CAD build for the part. Positions are in the model's coordinates, mm. Face numbers are marked on the shaded views. A direction names the side the tool comes from. Give positions to 0.01 mm unless a question says otherwise; leave off trailing zeros. Loops run counter-clockwise (first coordinate to the right, second up) from the corner with the lowest first, then second, coordinate; pieces in that order, holes last. Notation, with made-up numbers: M -21,63 L -17,63 A24 ccw -17,96 Z; hole C 70.25,-22 d3. An arc over 180 degrees is marked long. Answer as CSV lines item,"result".
from build123d import *

# Parameters (mm, degrees)
F1_DEPTH = 63.5
F2_DEPTH = 25.4
F3_DEPTH = 7.9375
F5_R     = 6.35


with BuildPart() as f1:
    # F0 (on Front) → F1 (new body, symmetric)
    with BuildSketch(Plane.XZ):
        Polygon((-46.0913150109, 34.0935156439), (-46.0913150109, 15.0435156439), (36.4586849891, 15.0435156439), (36.4586849891, 34.0935156439), (17.4086849891, 34.0935156439), align=None)
    extrude(amount=F1_DEPTH, both=True)

    # F0 (on Front) → F2 (join, symmetric)
    with BuildSketch(Plane.XZ):
        with BuildLine():
            Line((17.4086849891, 34.0935156439), (36.4586849891, 34.0935156439))
            Line((36.4586849891, 34.0935156439), (36.4586849891, 51.5687156439))
            ThreePointArc((36.4586849891, 51.5687156439), (41.1083648378, 62.7940357952), (52.3336849891, 67.4437156439))
            Line((52.3336849891, 67.4437156439), (55.9586890934, 67.4437156439))
            Line((55.9586890934, 67.4437156439), (55.9586890934, 86.4937156439))
            Line((55.9586890934, 86.4937156439), (52.3336849891, 86.4937156439))
            ThreePointArc((52.3336849891, 86.4937156439), (27.6379806562, 76.2644199768), (17.4086849891, 51.5687156439))
            Line((17.4086849891, 51.5687156439), (17.4086849891, 34.0935156439))
        make_face()
        Polygon((81.3586890934, 86.4937156439), (55.9586890934, 86.4937156439), (55.9586890934, 67.4437156439), (55.9586890934, 62.6685156439), (81.3586890934, 62.6685156439), align=None)
    extrude(amount=F2_DEPTH, both=True)

    # F0 (on Front) → F3 (join, symmetric)
    with BuildSketch(Plane.XZ):
        with BuildLine():
            add(Edge.make_bspline(
                [(-46.0913150109, 34.0935156439), (-45.8442233503, 68.7412694097), (0, 87.3479917645), (52.3336849891, 86.4937156439)],
                knots=[0, 0, 0, 0, 111.5045361635, 111.5045361635, 111.5045361635, 111.5045361635], degree=3))
            Line((-46.0913150109, 34.0935156439), (17.4086849891, 34.0935156439))
            Line((17.4086849891, 34.0935156439), (17.4086849891, 51.5687156439))
            ThreePointArc((17.4086849891, 51.5687156439), (27.6379806562, 76.2644199768), (52.3336849891, 86.4937156439))
        make_face()
    extrude(amount=F3_DEPTH, both=True)

    # F0 (on Front) → F4 (revolve)
    with BuildSketch(Plane.XZ):
        Polygon((81.3586890934, 91.2435156439), (81.3586890934, 86.4937156439), (81.3586890934, 62.6685156439), (106.7586890934, 62.6685156439), (106.7586890934, 91.2435156439), align=None)
    revolve(axis=Axis((81.3586890934, 0, 76.9560156439), (0, 0, -1)))

    # F5
    f5_edges = [f1.edges().sort_by_distance(p)[0] for p in [
        (36.458685, -63.5, 24.568516),
        (-46.091315, -63.5, 24.568516),
        (36.458685, 63.5, 24.568516),
        (-46.091315, 63.5, 24.568516),
    ]]
    fillet(f5_edges, radius=F5_R)


solid = f1.part
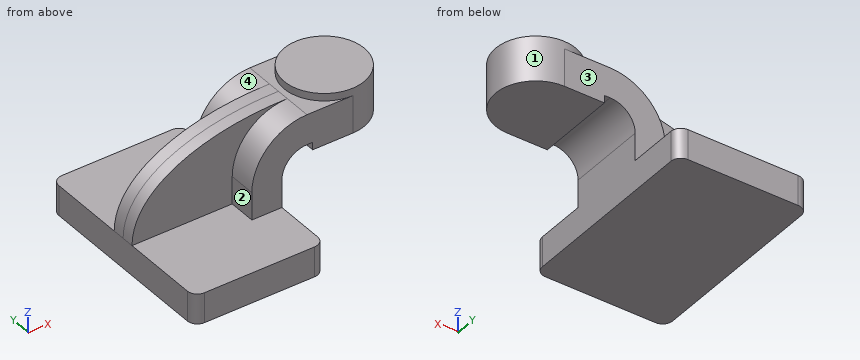
1) Drill centre lines: line 1 (Y direction, x = -16, z = 52.5); line 2 (X direction, y = 32, z = 25); line 3 (Z direction, x = 77.5, y = 17). Where is each one in solid material? Low to high. Write a range as from..to.
Answer below:
line 1,"y = -7.94..7.94"
line 2,"x = -46.09..36.46"
line 3,"z = 62.67..91.24"
2) Band-saw the part on C-C on x = 94.5. Give the cut face in (y, z).
Answer below:
outline,"M -21.74,62.67 L 21.74,62.67 L 21.74,91.24 L -21.74,91.24 Z"
3) Band-saw the part on B-B on y = 49.5. Give the cut face in (x, z).
Answer below:
outline,"M -46.09,15.04 L 36.46,15.04 L 36.46,34.09 L -46.09,34.09 Z"
4) Band-saw the part on A-A on x = 62. Give the cut face in (y, z), and give its area (3 significant figures).
Answer below:
outline,"M -25.4,62.67 L 25.4,62.67 L 25.4,86.49 L 16.44,86.49 L 16.44,91.24 L -16.44,91.24 L -16.44,86.49 L -25.4,86.49 Z"
area,"1,370 mm^2"
5) Which spindle directions (+Z, -Z, +X, -X, +Y, -Y) get a long thin tool onto all of the face, cutting with end or side? Do the marked faces 1, 2, 3 and 4. Say none if no direction does.
Answer below:
face 1,"+Z"
face 2,"+Z, -X, -Y"
face 3,"+Z, +X, -X, +Y"
face 4,"+Z, -X, +Y"
6) Flat gauge pins, fed straight in: pin 1 (3 mm diameter, centred on x = 13.5, y = 33.5, fed in from +Z); pin 2 (1.5 mm diameter, centred on x = 16.5, z = 83.5, fed in from -Y); pin 3 (5.5 mm diameter, centred on y = -3, z = 65, fed in from -X). Where does each tip first touch, or does it go through?
Answer below:
pin 1,"stops at z = 34.09"
pin 2,"stops at y = -7.94"
pin 3,"stops at x = -33.2"
